Check sheet for the modelled part. Datum: model origin and axes. Units: mm. A direction names the side the tool comes from. Round coordinates to 2 decimals unless told otherwise and drop trailing zeros. Loops run counter-clockwise (first coordinate to the right, second up) from the corner with the lowest first, then second, coordinate; pieces in that order, holes last. Notation, with made-up numbers: M -13.5,78 L 33.5,78 A25 cw 33.5,94 Z; hole C -31,51.5 d11. An arc over 180 degrees is marked long. Write item = value, one per line. Start each with the question number.
(1) Set-up check for faces 4 (the face through (0, 24, 12)), 5 (the face through (-6, -2, -2)), 6 (the face through (0, 0, 0)): record each of +Z, -Z, +X, -X, +Y, -Y from which the full face is reachable in a straight line by a thin tool's end or side.
(2) Go/stop test with flat-tipped pins: P1, Ø3, axis at x = -2.5, y = 18, coming from the +Z side; P2, Ø16, axis at x = -1.5, y = 40.5, coming from the +Z side; P3, Ø11, axis at x = 0, z = 0, coming from the -Y side; P4, Ø15.5, axis at x = 0, y = 39.894, coming from the -Z side. Record where each tip stops, or that it passes through.
(3) Cross-section at A-A on x = 0. Record the boundary of the cut face in (y, z).
(4) Cross-section at D-D on y = 43. Record the boundary of the cut face in (x, z).
(5) Cross-section at B-B on z = -20.5. Record the boundary of the cut face in (x, y).
(6) Cross-section at C-C on y = 15. Record the boundary of the cut face in (x, z), plus the area to 3 significant figures.
(7) Scan lines: L1, parallel to Y at x = 0.5, z = -21; L2, parallel to Y at x = 27, z = 12; L3, parallel to Y at x = 3, z = -7. Record each from-to range of solid material in increasing order. Write a range as from..to.
(8) Mould release check, pull along X, two halves, no side actions. Record for faces 1 (the face through (1.43, 21.3, -32.47)), 2 (the face through (3.23, 44.95, -16.02)), 3 (the face through (0, 47, 0)): pulls with the +X half, pulls with the -X half, needs draft (parallel to the pull), parting line crosses it, or undercut.
from build123d import *

# Parameters (mm, degrees)
SKETCH1_R           = 32.5
BOSS_EXTRUDE1_DEPTH = 55.788
CUT_EXTRUDE1_DEPTH  = 31.788
SKETCH3_R           = 8
SKETCH3_R_2         = 6
BOSS_EXTRUDE2_DEPTH = 2
SKETCH5_R           = 6
CUT_EXTRUDE3_DEPTH  = 46


with BuildPart() as part:
    # Sketch1 → Boss-Extrude1 (new body)
    with BuildSketch(Plane(origin=(0, 0, 0), x_dir=(1, 0, 0), z_dir=(0, 1, 0))):
        with Locations(Location((0, 0, 0), (0, 0, 270))):
            Circle(SKETCH1_R)
    extrude(amount=BOSS_EXTRUDE1_DEPTH)

    # Sketch2 → Cut-Extrude1 (cut)
    with BuildSketch(Plane(origin=(0, 55.788, 0), x_dir=(1, 0, 0), z_dir=(0, 1, 0))):
        with BuildLine():
            Line((32.5, 0), (-32.5, 0))
            ThreePointArc((-32.5, 0), (0, -32.5), (32.5, 0))
        make_face()
    extrude(amount=-CUT_EXTRUDE1_DEPTH, mode=Mode.SUBTRACT)

    # Sketch3 → Boss-Extrude2 (add)
    with BuildSketch(Plane(origin=(0, 0, 0), x_dir=(-1, 0, 0), z_dir=(0, -1, 0))):
        with Locations(Location((0, 0, 0), (0, 0, 270))):
            Circle(SKETCH3_R)
        with Locations(Location((0, 0, 0), (0, 0, 90))):
            Circle(SKETCH3_R_2, mode=Mode.SUBTRACT)
    extrude(amount=BOSS_EXTRUDE2_DEPTH)

    # Sketch5 → Cut-Extrude3 (cut)
    with BuildSketch(Plane.XY):
        with Locations((0, 39.894)):
            Circle(SKETCH5_R)
    extrude(amount=-CUT_EXTRUDE3_DEPTH, mode=Mode.SUBTRACT)


solid = part.part
Result:
q1.face_4 = +Z, +X, -X, +Y
q1.face_5 = +Z, -Z, +X, -X, -Y
q1.face_6 = -Y
q2.P1 = 32.48
q2.P2 = 0
q2.P3 = 0
q2.P4 = -32.5
q3.outline = M -2,-8 L 0,-8 L 0,-32.5 L 33.89,-32.5 L 33.89,0 L 24,0 L 24,32.5 L 0,32.5 L 0,8 L -2,8 L -2,6 L 0,6 L 0,-6 L -2,-6 Z; M 45.89,-32.5 L 55.79,-32.5 L 55.79,0 L 45.89,0 Z
q4.outline = M -32.5,0 A32.5 ccw -5.13,-32.09 L -5.13,0 Z; M 5.13,-32.09 A32.5 ccw 32.5,0 L 5.13,0 Z
q5.outline = M -25.22,0 L 25.22,0 L 25.22,55.79 L -25.22,55.79 Z; hole C 0,39.89 d12
q6.outline = C 0,0 d65
q6.area = 3,320 mm^2
q7.L1 = 0..33.91, 45.87..55.79
q7.L2 = 0..24
q7.L3 = -2..34.7, 45.09..55.79
q8.face_1 = parting line crosses it
q8.face_2 = undercut
q8.face_3 = needs draft
